Can you work these out from the model? Positions are in its coordinate system, mm. A direction names the side the tool comes from. Round coordinates to 2 decimals unless told otherwise and drop trailing zeros. Loops run counter-clockwise (first coordinate to the right, second up) from the corner with the lowest first, then second, coordinate; pieces in that order, holes last. Notation, with made-up numbers: (-3, 32.25) -> (35, 32.25) arc R7 cw to (35, 39.25) -> close; hole circle Ø1 at (89.25, 59.25). An arc over 180 degrees is marked (long way). Use a Markdown table: item, result.
Autodesk Inventor part; units mm, degrees
ref_plane "YZ Plane" through (0, 0, 0) normal (1, 0, 0) x (0, 1, 0)
ref_plane "XZ Plane" through (0, 0, 0) normal (0, 1, 0) x (-1, 0, 0)
ref_plane "XY Plane" through (0, 0, 0) normal (0, 0, 1) x (1, 0, 0)
sketch "Sketch1" plane through (0, 0, 0) normal (0, 1, 0) x (-1, 0, 0)
  circle A0 centre (0, 0) radius 5.2
  line L0 (1, 6.7) -> (-1, 6.7)
  line L1 (-1, 6.7) -> (-1, 3.7)
  line L2 (-1, 3.7) -> (1, 3.7)
  line L3 (1, 3.7) -> (1, 6.7)
  line L4 (1, 6.7) -> (-1, 3.7) construction
  line L5 (-1, 6.7) -> (1, 3.7) construction
  point P0 (0, 5.2)
  point P1 (1, 5.1029)
  point P2 (-1, 5.1029)
  dimension "d0" = 10.4
  dimension "d1" = 2
  dimension "d2" = 3
extrude "Extrusion1" add sketch "Sketch1" along normal blind 84.6 contours A0 L1 L2 L3 picked at (-0.1628, 0.741)
sketch "Sketch2" plane through (0, 84.6, 0) normal (0, 1, 0) x (1, 0, 0)
  circle A0 centre (0, 0) radius 1.45
  dimension "d5" = 2.9
extrude "Extrusion2" cut sketch "Sketch2" against normal blind 20
sketch "Sketch3" plane through (0, 0, 0) normal (0, -1, 0) x (1, 0, 0)
  circle A0 centre (0, 0) radius 1.45
extrude "Extrusion3" cut sketch "Sketch3" against normal blind 20
properties part number "00_Battery_AAA_Attrap"
1. If we mould it in two halves opening along Z, with no side actions, what happens to faces 1 (the flat face through (0, 64.6, 0)), 2 (the flat face through (1, 42, 4)), 3 (the cylindrical face through (-1.45, 9.86, 0.06)), 4 (the cylindrical face through (-0.215, 41.708, -5.196))? For each: +Z half, -Z half, draft (parallel to the pull), parting line (faces both ways), or undercut.
Answer sheet:
| item | result |
|---|---|
| face 1 | undercut |
| face 2 | draft |
| face 3 | undercut |
| face 4 | parting line |
2. I need wall thicknesses on line 1 (X direction, y = 71.25, z = 0); line 2 (Z direction, x = 0, y = 15.75); line 3 (X direction, y = 77.5, z = 4.75). Which ranges of each line are inside material? Lowest first, please.
Answer sheet:
| item | result |
|---|---|
| line 1 | x = -5.2 to -1.45, 1.45 to 5.2 |
| line 2 | z = -5.2 to -1.45, 1.45 to 3.7 |
| line 3 | x = -2.12 to -1, 1 to 2.12 |
3. I want a section at A-A (y = 17). Please give me the cut outline in (x, z), plus the area to 3 significant figures.
Answer sheet:
| item | result |
|---|---|
| outline | (-1, 3.7) -> (-1, 5.1) arc R5.2 ccw (long way) to (1, 5.1) -> (1, 3.7) -> close; hole circle Ø2.9 at (0, 0) |
| area | 75.4 mm² |
4. I want a section at D-D (y = 47). Please give me the cut outline in (x, z), plus the area to 3 significant figures.
Answer sheet:
| item | result |
|---|---|
| outline | (-1, 3.7) -> (-1, 5.1) arc R5.2 ccw (long way) to (1, 5.1) -> (1, 3.7) -> close |
| area | 82.0 mm² |
5. Will these pins go through, and if not, where does the flat tip stop? pin 1 Ø0.9 at (x, z) = (0, 0.5) entering from -Y; pin 2 Ø1.4 at (x, z) = (-0.5, -0.5) entering from +Y; pin 3 Ø1.5 at (y, z) = (21.5, 4) entering from +X.
Answer sheet:
| item | result |
|---|---|
| pin 1 | stops at y = 20 |
| pin 2 | stops at y = 64.6 |
| pin 3 | stops at x = 4.06 |
6. I want a section at B-B (z = 0). Please give me the cut outline in (x, y).
Answer sheet:
| item | result |
|---|---|
| outline | (-5.2, 0) -> (-1.45, 0) -> (-1.45, 20) -> (1.45, 20) -> (1.45, 0) -> (5.2, 0) -> (5.2, 84.6) -> (1.45, 84.6) -> (1.45, 64.6) -> (-1.45, 64.6) -> (-1.45, 84.6) -> (-5.2, 84.6) -> close |
7. I want a section at C-C (x = 0). Please give me the cut outline in (y, z).
Answer sheet:
| item | result |
|---|---|
| outline | (0, -5.2) -> (84.6, -5.2) -> (84.6, -1.45) -> (64.6, -1.45) -> (64.6, 1.45) -> (84.6, 1.45) -> (84.6, 3.7) -> (0, 3.7) -> (0, 1.45) -> (20, 1.45) -> (20, -1.45) -> (0, -1.45) -> close |
8. Which directions (+Z, -Z, +X, -X, +Y, -Y) give clear straight access to the entire face, cutting with the end or side of a thin tool? Please do faces 5 (the cylindrical face through (-1.45, 74.74, -0.06)), 6 (the flat face through (-1.1, 0, 1.2)), 7 (the flat face through (0, 42, 3.7)), 8 (the flat face through (0, 20, 0)), 9 (the flat face through (-1.1, 84.6, 1.2)).
Answer sheet:
| item | result |
|---|---|
| face 5 | +Y |
| face 6 | +Z, -Z, +X, -X, -Y |
| face 7 | +Z, +Y, -Y |
| face 8 | -Y |
| face 9 | +Z, -Z, +X, -X, +Y |
